Could you check a few things on this model? Use its own coordinates, in mm. A direction names the side the tool comes from. Give positions to 0.01 mm unless a question says otherwise; leave off trailing zeros. Write each loop counter-clockwise with the first axis right and the second up, starting at its lowest first coordinate (ties: lowest second). Pieces come first, ordered by that corner, then holes. Notation, with made-up numbers: M -11,5 L 19,5 A22 cw 19,18 Z; hole C 7.5,-12 d3. An arc over 180 degrees is marked long. Write each question's results on one line, items separated by ' | '. Start each with the question number.
from build123d import *

# Parameters (mm, degrees)
SKETCH_1_W           = 12.1
SKETCH_1_H           = 26
SKETCH_1_R           = 4.5
EXTRUDE_1_DEPTH      = 2.5
SKETCH_2_R           = 1.65
EXTRUDE_2_DEPTH      = 8
EXTRUDE_3_DEPTH      = 1
EXTRUDE_3_DEPTH_BACK = 3.5
SKETCH_3_R           = 5.25
SKETCH_3_R_2         = 4.5
FILLET_1_R           = 0.25


with BuildPart() as part:
    # Эскиз1 → Вытянуть1 (new body)
    with BuildSketch(Plane.XY):
        with Locations((0, 3)):
            Rectangle(SKETCH_1_W, SKETCH_1_H)
        Circle(SKETCH_1_R, mode=Mode.SUBTRACT)
    extrude(amount=EXTRUDE_1_DEPTH)

    # Эскиз2 → Вытянуть2 (add)
    with BuildSketch(Plane.XY.offset(2.5)):
        with Locations(Location((0, 10, 0), (0, 0, 180))):
            Circle(SKETCH_2_R)
    extrude(amount=EXTRUDE_2_DEPTH)

    # Эскиз3 → Вытянуть3 (add, two sides: drawn at the far end of the back side and taken through both)
    with BuildSketch(Plane.XY.offset(2.5).offset(-EXTRUDE_3_DEPTH_BACK)):
        Circle(SKETCH_3_R)
        Circle(SKETCH_3_R_2, mode=Mode.SUBTRACT)
    extrude(amount=EXTRUDE_3_DEPTH + EXTRUDE_3_DEPTH_BACK)

    # Скругление1
    fillet_1_edges = [part.edges().sort_by_distance(p)[0] for p in [
        (-4.5, 0, 3.5),
        (-5.25, 0, -1),
        (-4.5, 0, -1),
        (-5.25, 0, 3.5),
    ]]
    fillet(fillet_1_edges, radius=FILLET_1_R)


solid = part.part
Q1. If we section it at D-D (z = 8.5): Please give me the cut outline in (x, y), plus the area to 3 significant figures.
Q2. For faces 4 (the face through (6.05, 3, 1)), 5 (the face through (5, 1.6, -0.4)), 6 (the face through (5, 1.6, 2.9)), which set-ups out of +Z, -Z, +X, -X, +Y, -Y let a thin tool reach every point of the face, with its end or its side?
Q3. If we mould it in two halves opening along X, with no side actions, what happens to faces 1 (the face through (0.4, 11.6, 6.4)), 2 (the face through (0, -10, 1)), 3 (the face through (-0.59, 4.46, 1.22))? For each: pulls with the +X half, pulls with the -X half, needs draft (parallel to the pull), parting line crosses it, or undercut.
Q4. If we section it at A-A (y = 0): Please give me the cut outline in (x, z).
Q5. I'm going to push flat-ended pins straight in: P1, Ø1, axis at x = -1, z = 5, coming from the -Y side; P2, Ø3, axis at x = 4.5, y = 6, coming from the +Z side; P3, Ø4, axis at x = 1.5, z = 8, coming from the +Y side. Where does each tip first touch, or does it pass through?
Q6. Please list where these lines run through material, in increasing order: line 1 (Y direction, x = 0, z = 2.25); line 2 (Z direction, x = 0.75, y = 13.5); line 3 (Y direction, x = 3, z = 3.25). Write a range as [from, to].
Q7. If we section it at B-B (x = 0): Please give me the cut outline in (y, z), plus the area to 3 significant figures.
Q8. If we section it at C-C (y = 10.5): Please give me the cut outline in (x, z), plus the area to 3 significant figures.
Determined:
1) outline: C 0,10 d3.3 | area: 8.55 mm²
2) face 4: +Z, -Z, +X, +Y, -Y | face 5: -Z | face 6: +Z
3) face 1: parting line crosses it | face 2: needs draft | face 3: undercut
4) outline: M -6.05,0 L -5.25,0 L -5.25,-0.75 A0.25 ccw -5,-1 L -4.75,-1 A0.25 ccw -4.5,-0.75 L -4.5,3.25 A0.25 ccw -4.75,3.5 L -5,3.5 A0.25 ccw -5.25,3.25 L -5.25,2.5 L -6.05,2.5 Z; M 4.5,-0.75 A0.25 ccw 4.75,-1 L 5,-1 A0.25 ccw 5.25,-0.75 L 5.25,0 L 6.05,0 L 6.05,2.5 L 5.25,2.5 L 5.25,3.25 A0.25 ccw 5,3.5 L 4.75,3.5 A0.25 ccw 4.5,3.25 Z
5) P1: stops at y = 8.43 | P2: stops at z = 2.5 | P3: stops at y = 11.65
6) line 1: y = [-10, -4.5], [4.5, 16] | line 2: z = [0, 2.5] | line 3: y = [-4.31, -3.35], [3.35, 4.31]
7) outline: M -10,0 L -5.25,0 L -5.25,-0.75 A0.25 ccw -5,-1 L -4.75,-1 A0.25 ccw -4.5,-0.75 L -4.5,3.25 A0.25 ccw -4.75,3.5 L -5,3.5 A0.25 ccw -5.25,3.25 L -5.25,2.5 L -10,2.5 Z; M 4.5,-0.75 A0.25 ccw 4.75,-1 L 5,-1 A0.25 ccw 5.25,-0.75 L 5.25,0 L 16,0 L 16,2.5 L 11.65,2.5 L 11.65,10.5 L 8.35,10.5 L 8.35,2.5 L 5.25,2.5 L 5.25,3.25 A0.25 ccw 5,3.5 L 4.75,3.5 A0.25 ccw 4.5,3.25 Z | area: 71.8 mm²
8) outline: M -6.05,0 L 6.05,0 L 6.05,2.5 L 1.57,2.5 L 1.57,10.5 L -1.57,10.5 L -1.57,2.5 L -6.05,2.5 Z | area: 55.4 mm²
